from build123d import *

# Parameters (mm, degrees)
CROQUIS1_W              = 50.8
CROQUIS1_H              = 280
SALIENTE_EXTRUIR1_DEPTH = 12.7
CROQUIS2_W              = 24.610386892
CROQUIS2_H              = 50.8
SALIENTE_EXTRUIR2_DEPTH = 50
CROQUIS4_R              = 10.011889378
SALIENTE_EXTRUIR3_DEPTH = 100
CROQUIS5_W              = 7.310893966
CROQUIS5_H              = 140
CORTAR_EXTRUIR1_DEPTH   = 187.331823837


with BuildPart() as part:
    # Croquis1 → Saliente-Extruir1 (new body)
    with BuildSketch(Plane.XY):
        Rectangle(CROQUIS1_W, CROQUIS1_H)
    extrude(amount=SALIENTE_EXTRUIR1_DEPTH)

    # Croquis2 → Saliente-Extruir2 (add)
    with BuildSketch(Plane.XY.offset(12.7)):
        with Locations((-0.031570681, -114.6)):
            Rectangle(CROQUIS2_W, CROQUIS2_H)
    extrude(amount=SALIENTE_EXTRUIR2_DEPTH)

    # Croquis4 → Saliente-Extruir3 (add)
    with BuildSketch(Plane.ZY.offset(12.336764127)):
        with Locations(Location((41.7, -114.6, 0), (0, 0, 180))):
            Circle(CROQUIS4_R)
    extrude(amount=SALIENTE_EXTRUIR3_DEPTH)

    # Croquis5 → Cortar-Extruir1 (cut, through all)
    with BuildSketch(Plane.XY.offset(12.7)):
        with Locations((-21.744553017, -70)):
            Rectangle(CROQUIS5_W, CROQUIS5_H)
    extrude(amount=-CORTAR_EXTRUIR1_DEPTH, mode=Mode.SUBTRACT)


solid = part.part
Geometry check sheet. Reference: the model listing, model coordinates, mm. A direction names the side the tool comes from. Give positions to 0.01 mm unless a question says otherwise; leave off trailing zeros. Loops run counter-clockwise (first coordinate to the right, second up) from the corner with the lowest first, then second, coordinate; pieces in that order, holes last. Notation, with made-up numbers: (53, -32) -> (98, -32) arc R20 cw to (98, -5) -> close; hole circle Ø7 at (58.5, 0.25). An arc over 180 degrees is marked (long way). Answer in a Markdown table with one row per item. Add a question column.
1) Gauge pin test, flat ends, axial feed: P1, Ø15, axis at x = -9, y = -44.5, coming from the +Z side; P2, Ø6, axis at x = -35, z = 46.5, coming from the +Y side; P3, Ø14, axis at y = -61, z = 7, coming from the -X side. Record the tip position at first contact, or that the pin passes through.
2) Draft check along Z on faces 1 (the face through (0, -114, 62.7)), 2 (the face through (-18.089, -71, 6)), 3 (the face through (-12.337, -121, 32)), 4 (the face through (0, 2, 0)). Enter one of: pulls with the +Z half, pulls with the -Z half, needs draft (parallel to the pull), parting line crosses it, or undercut.
3) Set-up check for faces 5 (the face through (-22, 0, 6)), 6 (the face through (12.274, -115, 37)), 7 (the face through (-61.637, -123.042, 36.318)): record each of +Z, -Z, +X, -X, +Y, -Y from which the full face is reachable in a straight line by a thin tool's end or side.
4) Material ranges on probe 1 along Y at (x, z) = (-4, 42); probe 2 along X at (y, z) = (59, 6.5); probe 3 along Z at (x, y) = (-13.5, -72.5), recorded low to high. Write a range as from..to.
5) Cross-section at D-D on z = 8. Record the boundary of the cut face in (x, y).
6) Cross-section at B-B on z = 41.7. Record the boundary of the cut face in (x, y), and give its area (3 significant figures).
7) Cross-section at C-C on x = -99. Record the boundary of the cut face in (y, z).
8) Cross-section at A-A on y = -114.6. Record the boundary of the cut face in (x, z), and give its area (3 significant figures).
Outcome:
| question | item | result |
|---|---|---|
| 1 | P1 | stops at z = 12.7 |
| 1 | P2 | stops at y = -104.75 |
| 1 | P3 | stops at x = -18.09 |
| 2 | face 1 | pulls with the +Z half |
| 2 | face 2 | needs draft |
| 2 | face 3 | undercut |
| 2 | face 4 | pulls with the -Z half |
| 3 | face 5 | +Z, -Z, -X, -Y |
| 3 | face 6 | +Z, +X, +Y, -Y |
| 3 | face 7 | -X |
| 4 | probe 1 | y = -140..-89.2 |
| 4 | probe 2 | x = -25.4..25.4 |
| 4 | probe 3 | z = 0..12.7 |
| 5 | outline | (-25.4, 0) -> (-18.09, 0) -> (-18.09, -140) -> (25.4, -140) -> (25.4, 140) -> (-25.4, 140) -> close |
| 6 | outline | (-112.34, -124.61) -> (-12.34, -124.61) -> (-12.34, -140) -> (12.27, -140) -> (12.27, -89.2) -> (-12.34, -89.2) -> (-12.34, -104.59) -> (-112.34, -104.59) -> close |
| 6 | area | 3,250 mm^2 |
| 7 | outline | circle Ø20.02 at (-114.6, 41.7) |
| 8 | outline | (-112.34, 31.69) -> (-12.34, 31.69) -> (-12.34, 12.7) -> (-18.09, 12.7) -> (-18.09, 0) -> (25.4, 0) -> (25.4, 12.7) -> (12.27, 12.7) -> (12.27, 62.7) -> (-12.34, 62.7) -> (-12.34, 51.71) -> (-112.34, 51.71) -> close |
| 8 | area | 3,790 mm^2 |
